Geometry: final body of the model. Coordinates: model frame, mm. Face numbers are marked on the shaded views. A direction names the side the tool comes from. Give positions to 0.01 mm unless a question says otherwise; leave off trailing zeros. Write each loop counter-clockwise with the first axis right and the second up, starting at its lowest first coordinate (ties: lowest second). Pieces come first, ordered by that corner, then holes.
Q1. Line query: L1, parallel to Y at x = -11.7, z = 0; L2, parallel to X at y = -0.5, z = -9.5; L3, parallel to X at y = -2, z = -2. Output: solid intervals per line, ascending.
Q2. Cut plane D-D on x = 23. Return the cut outline in (y, z), plus the area to 3 significant figures.
Q3. Cut plane C-C on x = -8. Return the cut outline in (y, z).
Q4. Cut plane A-A on y = 0. Return the cut outline in (x, z).
Q5. Pin query (flat end, axial travel): pin 1 (5 mm diameter, centred on x = -10, z = -4, fed in from +Y); pin 2 (2 mm diameter, centred on y = -4, z = -5.5, fed in from -X); pin 3 (1.3 mm diameter, centred on x = -23, z = -0.5, fed in from +Y); pin 4 (10 mm diameter, centred on x = -16.5, y = 1.5, fed in from +Z). Return the tip coordinate at first contact, or that it passes through.
Q6. Reachability of the marked faces 1, 2 and 3 from +Z, -Z, +X, -X, +Y, -Y: full face, straight path, thin tool, end or side. Return the list, or none.
```python
from build123d import *

# Parameters (mm, degrees)
FILLET1_R          = 0.5
SKETCH2_W          = 8
SKETCH2_H          = 0.5
CUT_EXTRUDE1_DEPTH = 5
SKETCH3_R          = 1.5
CUT_EXTRUDE2_DEPTH = 5


with BuildPart() as part:
    # Sketch1 → Revolve1 (revolve)
    with BuildSketch(Plane.XY, mode=Mode.PRIVATE) as revolve1_sk:
        Polygon((-27, 0), (27, 0), (27, 12.1), (6.1, 12.1), (6, 12), (6, 12.5), (-15, 12.5), (-15, 3.5), (-17.5, 3.5), (-17.5, 2), (-27, 2), align=None)
    revolve(revolve1_sk.sketch.rotate(Axis((-27, 0, 0), (1, 0, 0)), 90), axis=Axis((-27, 0, 0), (1, 0, 0)))

    # Fillet1
    # the kernel refuses this fillet: 0.5 mm, written as the material it takes off along each edge
    with BuildSketch(Plane(origin=(27, 0, 0), x_dir=(0, 0, 1), z_dir=(0, 1, 0))) as fillet1_piece_1:
        with BuildLine():
            CenterArc((12.1 - FILLET1_R, -FILLET1_R), FILLET1_R, 0, 90)
            Line((12.1, -FILLET1_R), (12.1 + FILLET1_R * 0.02, -FILLET1_R))
            Line((12.1 + FILLET1_R * 0.02, -FILLET1_R), (12.1 + FILLET1_R * 0.02, FILLET1_R * 0.02))
            Line((12.1 + FILLET1_R * 0.02, FILLET1_R * 0.02), (12.1 - FILLET1_R, FILLET1_R * 0.02))
            Line((12.1 - FILLET1_R, FILLET1_R * 0.02), (12.1 - FILLET1_R, 0))
        make_face()
    revolve(axis=Axis((27, 0, 0), (1, 0, 0)), mode=Mode.SUBTRACT)
    with BuildSketch(Plane(origin=(6.1, 0, 0), x_dir=(0, 0, 1), z_dir=(0, 1, 0))) as fillet1_piece_2_section:
        with BuildLine():
            CenterArc((11.6, 0.2), FILLET1_R, 323.130102354, 36.869897646)
            Line((12, -0.1), (12.008, -0.106))
            ThreePointArc((12.008, -0.106), (12.057071068, -0.057071068), (12.107071068, -0.007071068))
            Line((12.107071068, -0.007071068), (12.11, 0))
            Line((12.11, 0), (12.11, 0.2))
            Line((12.11, 0.2), (12.1, 0.2))
        make_face()
    fillet1_piece_2 = revolve(axis=Axis((6.1, 0, 0), (1, 0, 0)), mode=Mode.PRIVATE)
    fillet1_piece_2 = split(fillet1_piece_2, bisect_by=Plane(origin=(6, 0, -12.082361586), z_dir=(1, 0, 0)), keep=Keep.TOP, mode=Mode.PRIVATE)
    add(fillet1_piece_2, mode=Mode.SUBTRACT)

    # Sketch2 → Cut-Extrude1 (cut, symmetric)
    with BuildSketch(Plane.XY):
        with Locations((-23, 1.75)):
            Rectangle(SKETCH2_W, SKETCH2_H)
    extrude(amount=CUT_EXTRUDE1_DEPTH, both=True, mode=Mode.SUBTRACT)

    # Sketch3 → Cut-Extrude2 (cut)
    with BuildSketch(Plane.ZY.offset(15)):
        with Locations((0, 8.5)):
            Circle(SKETCH3_R)
        with Locations((0, -8.5)):
            Circle(SKETCH3_R)
    extrude(amount=-CUT_EXTRUDE2_DEPTH, mode=Mode.SUBTRACT)


solid = part.part
```
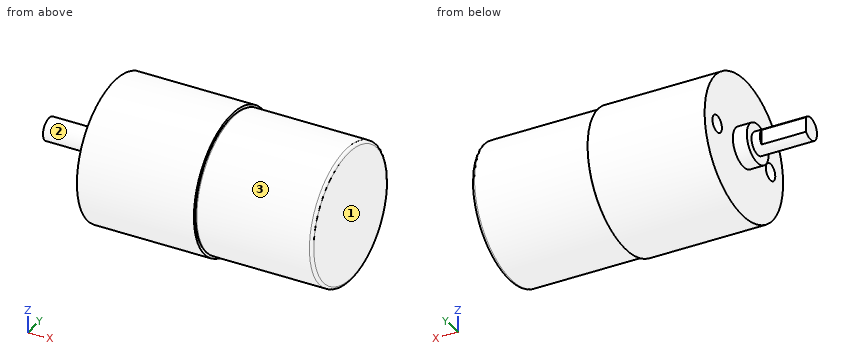
Data:
1. L1: y = -12.5 to -10, -7 to 7, 10 to 12.5
1. L2: x = -15 to 27
1. L3: x = -17.5 to 27
2. outline: circle Ø24.2 at (0, 0)
2. area: 460 mm2
3. outline: circle Ø25 at (0, 0)
4. outline: (-27, -2) - (-17.5, -2) - (-17.5, -3.5) - (-15, -3.5) - (-15, -12.5) - (6, -12.5) - (6, -12) arc R0.5 ccw to (6.3, -12.1) - (26.5, -12.1) arc R0.5 ccw to (27, -11.6) - (27, 11.6) arc R0.5 ccw to (26.5, 12.1) - (6.3, 12.1) arc R0.5 ccw to (6, 12) - (6, 12.5) - (-15, 12.5) - (-15, 3.5) - (-17.5, 3.5) - (-17.5, 2) - (-27, 2) - close
5. pin 1: stops at y = 12.41
5. pin 2: stops at x = -15
5. pin 3: stops at y = 1.5
5. pin 4: stops at z = 12.5
6. face 1: +Z, -Z, +X, +Y, -Y
6. face 2: -X
6. face 3: +X
